```python
from build123d import *

# Parameters (mm, degrees)
F2_ANGLE_BACK   = 5
F2_ANGLE        = 10
F2_COPIES_COUNT = 6
F3_SIZE         = 0.6


# Not quite as in the source:
# - a pattern or mirror of a feature is missing from the dataset's text; its kind, count and spacing are read off the source's solid


with BuildPart() as f1:
    # F0 (on Front) → F1 (revolve)
    with BuildSketch(Plane.XZ):
        Polygon((-2, 0), (0, 0), (0, 11), (-2, 11), (-2, 10.25), (-2, 9.5), (-17, 9.5), (-17, 7), (-2, 7), align=None)
    revolve(axis=Axis((-8.5, 0, 0), (-1, 0, 0)))

    # F0 (on Front) → F2 (revolve)
    with BuildSketch(Plane.XZ, mode=Mode.PRIVATE) as f2_sk:
        Polygon((-2, 9.5), (-2, 10.25), (-12, 10.25), (-17, 9.5), align=None)
    f2 = revolve(f2_sk.sketch.rotate(Axis((-8.5, 0, 0), (-1, 0, 0)), -F2_ANGLE_BACK), axis=Axis((-8.5, 0, 0), (-1, 0, 0)), revolution_arc=F2_ANGLE)

    # F2_copies: F2 ×6 about axis
    f2_copies_axis = Axis((0, 0, 0), (1, 0, 0))
    for i in range(1, F2_COPIES_COUNT):
        add(f2.rotate(f2_copies_axis, i * 360 / F2_COPIES_COUNT))

    # F3
    f3_edges = [f1.edges().sort_by_distance(p)[0] for p in [
        (0, 0, -11),
    ]]
    chamfer(f3_edges, length=F3_SIZE)


solid = f1.part
```
Source: CAD feature listing. Evaluate the final solid. Frame: model axes, mm. A direction names the side the tool comes from. Round coordinates to 2 decimals unless told otherwise and drop trailing zeros. Order: outer loops, then holes, each group sorted by start corner. A loop starts at its lowest first (then second) coordinate and runs counter-clockwise, first axis right, second up. Notation, with made-up numbers: (23, 4.5) -> (44, 4.5) arc R26 ccw to (44, 41.5) -> close; hole circle Ø9 at (-37, 10). An arc over 180 degrees is marked (long way). Use CSV: the item, a comma, the result in double quotes.
(1) Pull-direction query (Y, two-part tool) for faces 1 (the face through (-7.07, -8.87, -5.14)), 2 (the face through (-9.395, -2.681, 6.466)), 3 (the face through (-14.54, 8.54, 4.95)); classes: +Y half, -Y half, draft (parallel to the pull), parting line (faces both ways), or undercut.
Report:
face 1,"-Y half"
face 2,"undercut"
face 3,"+Y half"
(2) Section B-B on y = 0. Return the cut outline in (x, z).
Report:
outline,"(-17, -9.5) -> (-12, -10.25) -> (-2, -10.25) -> (-2, -11) -> (-0.6, -11) -> (0, -10.4) -> (0, 10.4) -> (-0.6, 11) -> (-2, 11) -> (-2, 10.25) -> (-12, 10.25) -> (-17, 9.5) -> (-17, 7) -> (-2, 7) -> (-2, -7) -> (-17, -7) -> close"
(3) Ray query, L1, parallel to Y at x = -7, z = 0; L2, parallel to X at y = -3, z = -5.25; L3, parallel to Z at x = -2.25, y = -1.5. Return the intervals inside material, ascending.
Report:
L1,"-9.5 to -7, 7 to 9.5"
L2,"-2 to 0"
L3,"-9.38 to -6.84, 6.84 to 9.38"
(4) Access query for faces 4 (the face through (-7.07, 0.01, -10.25)), 5 (the face through (-7.07, 8.87, 5.14)), 6 (the face through (-9.6, 9.5, 0.1)), 7 (the face through (-7.07, 8.883, -5.114)), 8 (the face through (-2, 0, 0)). Directions: +Z, -Z, +X, -X, +Y, -Y. A direction counts if a zero-diameter tool reaches every point of the face in a straight line with its end or side. Return the directions, or none.
Report:
face 4,"-Z, -X"
face 5,"+Z, -X, +Y"
face 6,"-X, +Y"
face 7,"-Z, -X, +Y"
face 8,"-X"
(5) Section C-C on z = 0. Return the cut outline in (x, y), and give its area (3 significant figures).
Report:
outline,"(-17, -9.5) -> (-2, -9.5) -> (-2, -11) -> (-0.6, -11) -> (0, -10.4) -> (0, 10.4) -> (-0.6, 11) -> (-2, 11) -> (-2, 9.5) -> (-17, 9.5) -> (-17, 7) -> (-2, 7) -> (-2, -7) -> (-17, -7) -> close"
area,"119 mm^2"
(6) First-contact query: pin 1 Ø2 at (x, y) = (-7.5, 0.5) entering from +Z; pin 2 Ø1.5 at (x, z) = (-8, -4.5) entering from -Y; pin 3 Ø4 at (x, y) = (-9, -3) entering from +Z. Flat tips, straight axial feed; report the tip coordinate or a pass-through.
Report:
pin 1,"z = 10.25"
pin 2,"y = -9.29"
pin 3,"z = 9.45"
(7) Section A-A on x = -11.25. Return the cut outline in (y, z), and give its area (3 significant figures).
Report:
outline,"(-9.29, -4.33) arc R10.25 ccw to (-8.4, -5.88) -> (-7.78, -5.45) arc R9.5 ccw to (-0.83, -9.46) -> (-0.89, -10.21) arc R10.25 ccw to (0.89, -10.21) -> (0.83, -9.46) arc R9.5 ccw to (7.78, -5.45) -> (8.4, -5.88) arc R10.25 ccw to (9.29, -4.33) -> (8.61, -4.01) arc R9.5 ccw to (8.61, 4.01) -> (9.29, 4.33) arc R10.25 ccw to (8.4, 5.88) -> (7.78, 5.45) arc R9.5 ccw to (0.83, 9.46) -> (0.89, 10.21) arc R10.25 ccw to (-0.89, 10.21) -> (-0.83, 9.46) arc R9.5 ccw to (-7.78, 5.45) -> (-8.4, 5.88) arc R10.25 ccw to (-9.29, 4.33) -> (-8.61, 4.01) arc R9.5 ccw to (-8.61, -4.01) -> close; hole circle Ø14 at (0, 0)"
area,"137 mm^2"
